Geometry check sheet. Reference: drawing and pictorial views, mm from the part's lowest x, y, z. A direction names the side the tool comes from. Give positions to 0.01 mm unless a question says otherwise; leave off trailing zeros. Write each loop counter-clockwise with the first axis right and the second up, starting at its lowest first coordinate (ties: lowest second). Pieces come first, ordered by that corner, then holes. Notation, with made-up numbers: M 71.5,61 L 80.5,61 A33 ccw 80.5,97 Z; hole C 13.5,13 d11. An arc over 180 degrees is marked long. One line per item, written item: value. Start each with the question number.
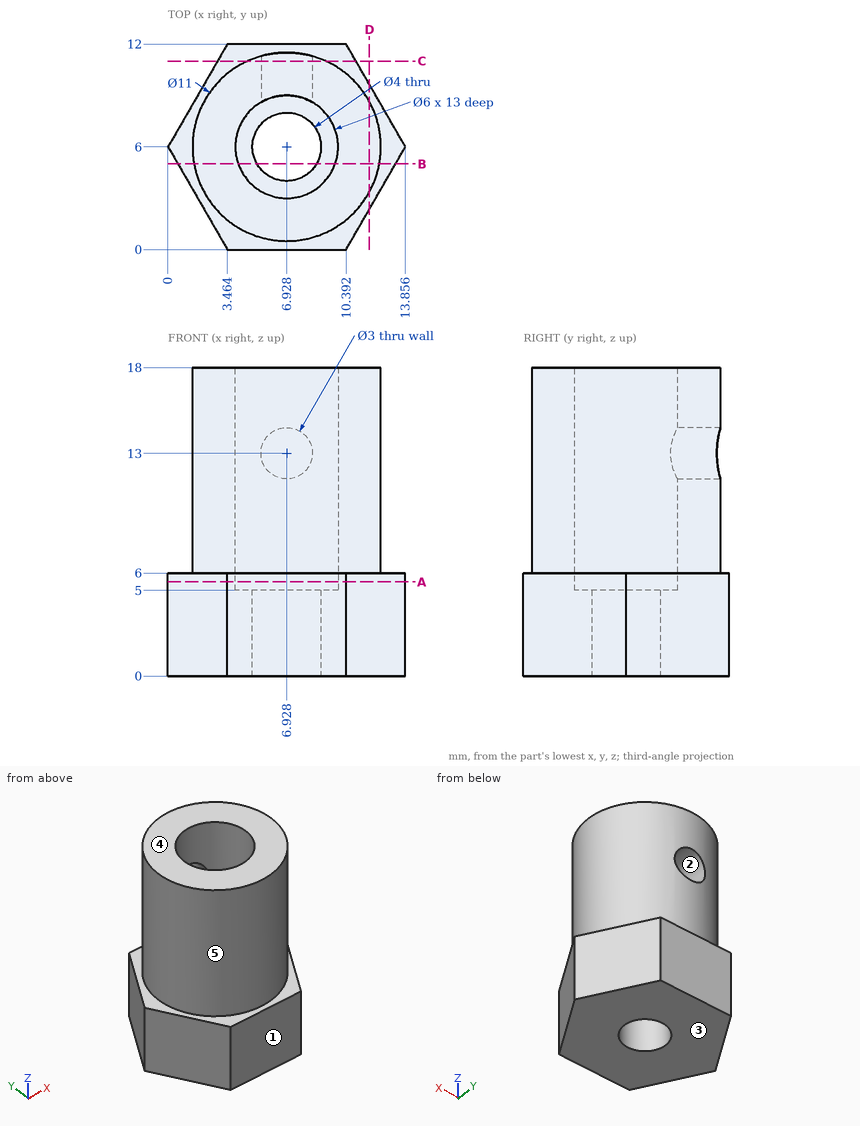
1) Draft check along Z on the marked faces 1, 2 and 3. Enter one of: released by +Z, released by -Z, zero draft, split by the parting line, or undercut.
2) Gauge pin test, flat ends, axial feed: pin 1 (6 mm diameter, centred on y = 6, z = 16, fed in from +X); pin 2 (1.8 mm diameter, centred on x = 6.93, z = 13, fed in from +Y); pin 3 (3 mm diameter, centred on x = 8.5, z = 11.5, fed in from -Y). Record the tip position at first contact, or that the pin passes through.
3) Cross-section at A-A (z = 5.5). Record the boundary of the cut face in (x, y).
4) Cross-section at D-D (x = 11.75). Record the boundary of the cut face in (y, z) (1 decimal).
5) Cross-section at C-C (y = 11). Record the boundary of the cut face in (x, z).
6) Cross-section at B-B (y = 5). Record the boundary of the cut face in (x, z).
7) Tool access check on the marked faces 4 and 5. Record the directions out of +Z, -Z, +X, -X, +Y, -Y that give a thin tool (end or side, any length) a straight path to the whole face; none if there is none.
8) Material ranges on L1, parallel to Z at x = 7.75, y = 3.5; L2, parallel to Y at x = 7, z = 17.25; L3, parallel to Z at x = 4.5, y = 11, recorded low to high. Write a range as from..to.
Data:
1. face 1: zero draft
1. face 2: undercut
1. face 3: released by -Z
2. pin 1: stops at x = 12.43
2. pin 2: stops at y = 3.14
2. pin 3: stops at y = 0.5
3. outline: M 0,6 L 3.46,0 L 10.39,0 L 13.86,6 L 10.39,12 L 3.46,12 Z; hole C 6.93,6 d6
4. outline: M 2.4,0 L 9.6,0 L 9.6,6 L 8.6,6 L 8.6,18 L 3.4,18 L 3.4,6 L 2.4,6 Z
5. outline: M 2.89,0 L 10.97,0 L 10.97,6 L 9.22,6 L 9.22,18 L 4.64,18 L 4.64,6 L 2.89,6 Z; hole C 6.93,13 d3
6. outline: M 0.58,0 L 5.2,0 L 5.2,5 L 4.1,5 L 4.1,18 L 1.52,18 L 1.52,6 L 0.58,6 Z; M 8.66,0 L 13.28,0 L 13.28,6 L 12.34,6 L 12.34,18 L 9.76,18 L 9.76,5 L 8.66,5 Z
7. face 4: +Z, +X, -X, +Y, -Y
7. face 5: +Z
8. L1: z = 0..5
8. L2: y = 0.5..3, 9..11.5
8. L3: z = 0..6
